```python
from build123d import *

# Parameters (mm, degrees)
F0_W      = 58
F0_H      = 10
F0_R      = 2
F1_DEPTH  = 4
F2_W      = 29
F2_H      = 10
F3_DEPTH  = 4
F4_W      = 15
F4_H      = 10
F5_DEPTH  = 4
F6_DEPTH  = 12
F7_W      = 29
F7_H      = 11
F8_DEPTH  = 6
F9_W      = 29
F9_H      = 11
F9_W_2    = 13
F10_DEPTH = 4
F11_R     = 2
F12_DEPTH = 4


with BuildPart() as f1:
    # F0 (on Front) → F1 (new body)
    with BuildSketch(Plane.XZ):
        Rectangle(F0_W, F0_H)
        with Locations((-20, 0)):
            Circle(F0_R, mode=Mode.SUBTRACT)
        with BuildLine():
            ThreePointArc((22, 0), (20, -2), (18, 0))
            ThreePointArc((18, 0), (20, 2), (22, 0))
        make_face(mode=Mode.SUBTRACT)
    extrude(amount=F1_DEPTH)

    # F2 (on face) → F3 (join)
    with BuildSketch(Plane(origin=(0, 0, 0), x_dir=(-1, 0, 0), z_dir=(0, 1, 0))):
        Rectangle(F2_W, F2_H)
    extrude(amount=F3_DEPTH)

    # F4 (on face) → F5 (cut)
    with BuildSketch(Plane.XZ.offset(4)):
        Rectangle(F4_W, F4_H)
    extrude(amount=-F5_DEPTH, mode=Mode.SUBTRACT)

    # F6 (add): a face of the model
    f6_faces = [f1.faces().sort_by_distance(p)[0] for p in [
        (-21.75, -0.5854912467, -5),
    ]]
    extrude(f6_faces, amount=F6_DEPTH)

    # F7 (on face) → F8 (join)
    with BuildSketch(Plane(origin=(0, 4, 0), x_dir=(-1, 0, 0), z_dir=(0, 1, 0))):
        with Locations((0, -11.5)):
            Rectangle(F7_W, F7_H)
    extrude(amount=F8_DEPTH)

    # F9 (on face) → F10 (join)
    with BuildSketch(Plane(origin=(0, 10, 0), x_dir=(-1, 0, 0), z_dir=(0, 1, 0))):
        with Locations((0, -11.5)):
            Rectangle(F9_W, F9_H)
        with Locations((-21, -11.5)):
            Rectangle(F9_W_2, F9_H)
        with Locations((21, -11.5)):
            Rectangle(F9_W_2, F9_H)
    extrude(amount=F10_DEPTH)

    # F11 (on face) → F12 (cut)
    with BuildSketch(Plane(origin=(0, 14, 0), x_dir=(-1, 0, 0), z_dir=(0, 1, 0))):
        with Locations((-21.5, -11.5)):
            Circle(F11_R)
        with BuildLine():
            ThreePointArc((23.5, -11.5), (21.5, -9.5), (19.5, -11.5))
            ThreePointArc((19.5, -11.5), (21.5, -13.5), (23.5, -11.5))
        make_face()
    extrude(amount=-F12_DEPTH, mode=Mode.SUBTRACT)


solid = f1.part
```
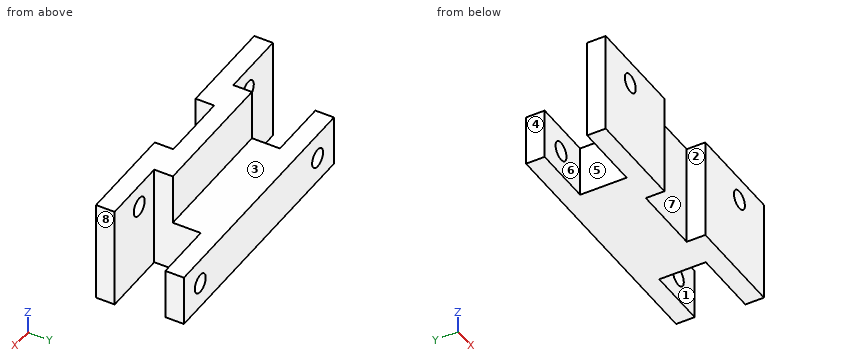
Input: part model. Units: mm. Frame: model coordinates. Face numbers are marked on the shaded views. A direction names the side the tool comes from. Give positions to 0.01 mm unless a question says otherwise; leave off trailing zeros. Write each loop counter-clockwise with the first axis right and the second up, starting at its lowest first coordinate (ties: lowest second). Pieces come first, ordered by that corner, then holes. Notation, with made-up numbers: (10.25, 55.5) - (38.25, 55.5) arc R18 cw to (38.25, 87.5) - close; hole circle Ø3 at (-21, -36). An arc over 180 degrees is marked (long way). Write item = value, one per line. Start each with the question number.
1) Cut plane B-B (x = 21). Return loops of the section in (y, z).
2) Draft query along X for the marked faces 6, 7 and 8. Return one class per face: pulls with the +X half, pulls with the -X half, needs draft (parallel to the pull), parting line crosses it, or undercut.
3) Cut plane C-C (z = -11.5). Return loops of the section in (x, y).
4) Pin query (flat end, axial travel): pin 1 (3 mm diameter, centred on x = 21.5, z = -11.5, fed in from +Y); pin 2 (3 mm diameter, centred on x = -6.5, y = 7.5, fed in from +Z); pin 3 (1.5 mm diameter, centred on y = 8, z = -13, fed in from +X). Return the tip coordinate at first contact, or that it passes through.
5) Reachability of the marked faces 1, 2, 3, 4 and 5 from +Z, -Z, +X, -X, +Y, -Y: full face, straight path, thin tool, end or side. Return the list, or none.
6) Cut plane D-D (y = 6). Return loops of the section in (x, z).
7) Cut plane A-A (z = 0). Return loops of the section in (x, y).
8) Material intervals for L1, parallel to X at y = -0.75, z = -15; L2, parallel to Z at x = -21.5, y = 13.15; L3, parallel to Y at x = -16.5, z = -13.5, sorted ascending. Write a range as [from, to].
Answers follow:
q1.outline = (-4, -17) - (0, -17) - (0, -1.73) - (-4, -1.73) - close; (-4, 1.73) - (0, 1.73) - (0, 5) - (-4, 5) - close; (10, -17) - (14, -17) - (14, -13.44) - (10, -13.44) - close; (10, -9.56) - (14, -9.56) - (14, -6) - (10, -6) - close
q2.face_6 = needs draft
q2.face_7 = undercut
q2.face_8 = pulls with the +X half
q3.outline = (-29, -4) - (-7.5, -4) - (-7.5, 0) - (7.5, 0) - (7.5, -4) - (29, -4) - (29, 0) - (14.5, 0) - (14.5, 10) - (19.5, 10) - (19.5, 14) - (-19.5, 14) - (-19.5, 10) - (-14.5, 10) - (-14.5, 0) - (-29, 0) - close; (-27.5, 10) - (-23.5, 10) - (-23.5, 14) - (-27.5, 14) - close; (23.5, 10) - (27.5, 10) - (27.5, 14) - (23.5, 14) - close
q4.pin_1 = 0
q4.pin_2 = -6
q4.pin_3 = 14.5
q5.face_1 = +Z, -Z, +X
q5.face_2 = +Z, -Z, -Y
q5.face_3 = +Z, +X, -X, +Y
q5.face_4 = +Z, -Z, -X, +Y
q5.face_5 = +Z, -Z, -X
q6.outline = (-14.5, -17) - (14.5, -17) - (14.5, -6) - (-14.5, -6) - close
q7.outline = (-29, -4) - (-22, -4) - (-22, 0) - (-29, 0) - close; (-18, -4) - (-7.5, -4) - (-7.5, 0) - (7.5, 0) - (7.5, -4) - (18, -4) - (18, 0) - (14.5, 0) - (14.5, 4) - (-14.5, 4) - (-14.5, 0) - (-18, 0) - close; (22, -4) - (29, -4) - (29, 0) - (22, 0) - close
q8.L1 = [-29, -7.5], [7.5, 29]
q8.L2 = [-17, -13.5], [-9.5, -6]
q8.L3 = [-4, 0], [10, 14]
